from build123d import *

# Parameters (mm, degrees)
SKETCH1_W                 = 130
SKETCH1_H                 = 125
BOSS_EXTRUDE1_DEPTH       = 3
SKETCH2_R                 = 1.75
SKETCH2_R_2               = 12.65
CUT_EXTRUDE1_DEPTH        = 10
MIRROR4_COPY_1_SKETCH_R   = 1.75
MIRROR4_COPY_1_SKETCH_R_2 = 12.65
MIRROR4_COPY_1_DEPTH      = 10
SKETCH3_R                 = 2.65
CUT_EXTRUDE2_DEPTH        = 10
SKETCH4_R                 = 2.65
CUT_EXTRUDE3_DEPTH        = 10


with BuildPart() as part:
    # Sketch1 → Boss-Extrude1 (new body)
    with BuildSketch(Plane(origin=(0, 0, 0), x_dir=(1, 0, 0), z_dir=(0, 1, 0))):
        Rectangle(SKETCH1_W, SKETCH1_H)
    extrude(amount=BOSS_EXTRUDE1_DEPTH)

    # Sketch2 → Cut-Extrude1 (cut)
    with BuildSketch(Plane(origin=(0, 3, 0), x_dir=(1, 0, 0), z_dir=(0, 1, 0))):
        with Locations(Location((-61, -52.5, 0), (0, 0, 270))):
            Circle(SKETCH2_R)
        with Locations(Location((-36, -52.5, 0), (0, 0, 270))):
            Circle(SKETCH2_R)
        with Locations(Location((-36, -10.5, 0), (0, 0, 270))):
            Circle(SKETCH2_R)
        with Locations(Location((-61, -10.5, 0), (0, 0, 270))):
            Circle(SKETCH2_R)
        with Locations(Location((-45.5, -31.5, 0), (0, 0, 270))):
            Circle(SKETCH2_R_2)
    cut_extrude1 = extrude(amount=-CUT_EXTRUDE1_DEPTH, mode=Mode.SUBTRACT)

    # Mirror3: Cut-Extrude1 across plane
    add(cut_extrude1.mirror(Plane.ZY), mode=Mode.SUBTRACT)

    # Mirror4: Cut-Extrude1 across plane
    add(cut_extrude1.mirror(Plane.XY), mode=Mode.SUBTRACT)

    # Mirror4 copy 1 sketch → Mirror4 copy 1 (cut)
    with BuildSketch(Plane(origin=(0, 3, 0), x_dir=(-1, 0, 0), z_dir=(0, 1, 0))):
        with Locations(Location((-61, -52.5, 0), (0, 0, 270))):
            Circle(MIRROR4_COPY_1_SKETCH_R)
        with Locations(Location((-36, -52.5, 0), (0, 0, 270))):
            Circle(MIRROR4_COPY_1_SKETCH_R)
        with Locations(Location((-36, -10.5, 0), (0, 0, 270))):
            Circle(MIRROR4_COPY_1_SKETCH_R)
        with Locations(Location((-61, -10.5, 0), (0, 0, 270))):
            Circle(MIRROR4_COPY_1_SKETCH_R)
        with Locations(Location((-45.5, -31.5, 0), (0, 0, 270))):
            Circle(MIRROR4_COPY_1_SKETCH_R_2)
    extrude(amount=-MIRROR4_COPY_1_DEPTH, mode=Mode.SUBTRACT)

    # Sketch3 → Cut-Extrude2 (cut)
    with BuildSketch(Plane(origin=(0, 3, 0), x_dir=(1, 0, 0), z_dir=(0, 1, 0))):
        with Locations(Location((-24.17, -42.03, 0), (0, 0, 270))):
            Circle(SKETCH3_R)
        with Locations(Location((24.17, -42.03, 0), (0, 0, 270))):
            Circle(SKETCH3_R)
        with Locations(Location((-8.73, 9.6, 0), (0, 0, 270))):
            Circle(SKETCH3_R)
        with Locations(Location((19.29, 9.6, 0), (0, 0, 270))):
            Circle(SKETCH3_R)
        with Locations(Location((-24.17, 33.11, 0), (0, 0, 270))):
            Circle(SKETCH3_R)
        with Locations(Location((24.17, 40.6, 0), (0, 0, 270))):
            Circle(SKETCH3_R)
    extrude(amount=-CUT_EXTRUDE2_DEPTH, mode=Mode.SUBTRACT)

    # Sketch4 → Cut-Extrude3 (cut)
    with BuildSketch(Plane(origin=(0, 3, 0), x_dir=(1, 0, 0), z_dir=(0, 1, 0))):
        with Locations(Location((0, 47.5, 0), (0, 0, 270))):
            Circle(SKETCH4_R)
        with Locations(Location((12.049810205, 55, 0), (0, 0, 270))):
            Circle(SKETCH4_R)
        with Locations(Location((-12.049810205, 55, 0), (0, 0, 270))):
            Circle(SKETCH4_R)
    extrude(amount=-CUT_EXTRUDE3_DEPTH, mode=Mode.SUBTRACT)


solid = part.part
Could you check a few things on this model? Use its own coordinates, in mm. Give positions to 0.01 mm unless a question says otherwise; leave off trailing zeros. Order: outer loops, then holes, each group sorted by start corner. A loop starts at its lowest first (then second) coordinate and runs counter-clockwise, first axis right, second up.
Item 1: If we section it at C-C, the plane z = 31.5: Write out the boundary of the cut face in (x, y), plus the area to 3 significant figures.
Item 2: I need wall thicknesses on line 1 (X direction, y = 2.15, z = -55); line 2 (X direction, y = 0.8, z = 52.5); line 3 (X direction, y = 0.35, z = 23). Which ranges of each line are inside material? Lowest first, please.
Item 3: I'm going to push a flat-ended pin straight in: pin 1 (3 mm diameter, centred on x = -36, z = -10.5, fed in from -Y). Where does the tip first touch, or does it pass through?
Item 4: If we section it at B-B, the plane z = 52.5: Write out the boundary of the cut face in (x, y).
Item 5: If we section it at A-A, the plane x = 45.5: Write out the boundary of the cut face in (y, z).
Item 6: If we section it at D-D, the plane y = 0.7: Count the separate pieces of the cut face and the enclosed holes in it, plus the area to 3 significant figures.
Item 7: If we mould it in two halves opening along X, with no side actions, what happens to faces 1 (the face through (-65, 1, 1)), 2 (the face through (-1, 0, -1)), 3 (the face through (0.117, 1.521, -50.147))? For each: pulls with the +X half, pulls with the -X half, needs draft (parallel to the pull), parting line crosses it, or undercut.
Values:
1. outline: (-65, 0) - (-58.15, 0) - (-58.15, 3) - (-65, 3) - close; (-32.85, 0) - (32.85, 0) - (32.85, 3) - (-32.85, 3) - close; (58.15, 0) - (65, 0) - (65, 3) - (58.15, 3) - close
1. area: 238 mm2
2. line 1: x = -65 to -14.7, -9.4 to 9.4, 14.7 to 65
2. line 2: x = -65 to -62.75, -59.25 to -37.75, -34.25 to 34.25, 37.75 to 59.25, 62.75 to 65
2. line 3: x = -65 to -54.87, -36.13 to 36.13, 54.87 to 65
3. pin 1: passes through
4. outline: (-65, 0) - (-62.75, 0) - (-62.75, 3) - (-65, 3) - close; (-59.25, 0) - (-37.75, 0) - (-37.75, 3) - (-59.25, 3) - close; (-34.25, 0) - (34.25, 0) - (34.25, 3) - (-34.25, 3) - close; (37.75, 0) - (59.25, 0) - (59.25, 3) - (37.75, 3) - close; (62.75, 0) - (65, 0) - (65, 3) - (62.75, 3) - close
5. outline: (0, -62.5) - (3, -62.5) - (3, -44.15) - (0, -44.15) - close; (0, -18.85) - (3, -18.85) - (3, 18.85) - (0, 18.85) - close; (0, 44.15) - (3, 44.15) - (3, 62.5) - (0, 62.5) - close
6. separate pieces: 1
6. enclosed holes: 29
6. area: 13,900 mm2
7. face 1: pulls with the -X half
7. face 2: needs draft
7. face 3: undercut
